Geometry check sheet. Reference: the model listing, model coordinates, mm. A direction names the side the tool comes from. Give positions to 0.01 mm unless a question says otherwise; leave off trailing zeros. Write each loop counter-clockwise with the first axis right and the second up, starting at its lowest first coordinate (ties: lowest second). Pieces come first, ordered by that corner, then holes.
(1) Cross-section at B-B (y = 0). Record the boundary of the cut face in (x, z), and give its area (3 significant figures).
(2) Cross-section at C-C (z = 4.5). Record the boundary of the cut face in (x, y).
(3) Tool access check on faces 1 (the flat face through (124.627, -15, 25)), 2 (the flat face through (-2, 83.745, 25)). Record the directions out of +Z, -Z, +X, -X, +Y, -Y that give a thin tool (end or side, any length) a straight path to the whole face; none if there is none.
(4) Mould release check, pull along X, two halves, no side actions. Record for faces 3 (the flat face through (121.627, -12, 25)), 4 (the flat face through (-125.373, -12, 25)), 5 (the flat face through (-2, -110.255, 25)), 6 (the flat face through (1, 86.745, 25)): +X half, -X half, draft (parallel to the pull), parting line (faces both ways), or undercut.
(5) Thickness scan on line 1 along X through (y, z) = (-99.5, 46); line 2 along Y through (x, z) = (18, 35). Record the ranges inside material, lowest first.
(6) Cross-section at A-A (x = -89). Record the boundary of the cut face in (y, z).
```python
from build123d import *

# Parameters (mm, degrees)
F0_W     = 3
F0_H     = 97
F0_H_2   = 3
F0_W_2   = 122
F0_W_3   = 115.3171807528
F0_W_4   = 6.6828192472
F0_W_5   = 244
F1_DEPTH = 50


with BuildPart() as f1:
    # F0 (on Top) → F1 (new body)
    with BuildSketch(Plane.XY):
        with Locations((-123.8728196025, 35.2448651371)):
            Rectangle(F0_W, F0_H)
        with Locations((-123.8728196025, 85.2448651371)):
            Rectangle(F0_W, F0_H_2)
        with Locations((-61.3728196025, 85.2448651371)):
            Rectangle(F0_W_2, F0_H_2)
        with Locations((57.2857707739, 85.2448651371)):
            Rectangle(F0_W_3, F0_H_2)
        with Locations((118.2857707739, 85.2448651371)):
            Rectangle(F0_W_4, F0_H_2)
        with Locations((123.1271803975, 85.2448651371)):
            Rectangle(F0_W, F0_H_2)
        Polygon((124.6271803975, 83.7448651371), (121.6271803975, 83.7448651371), (121.6271803975, -110.2551348629), (121.6271803975, -113.2551348629), (124.6271803975, -113.2551348629), align=None)
        with Locations((-0.3728196025, -111.7551348629)):
            Rectangle(F0_W_5, F0_H_2)
        with Locations((-123.8728196025, -61.7551348629)):
            Rectangle(F0_W, F0_H)
        with Locations((-123.8728196025, -111.7551348629)):
            Rectangle(F0_W, F0_H_2)
    extrude(amount=F1_DEPTH)


solid = f1.part
```
Reply:
1. outline: (-125.37, 0) - (-122.37, 0) - (-122.37, 50) - (-125.37, 50) - close; (121.63, 0) - (124.63, 0) - (124.63, 50) - (121.63, 50) - close
1. area: 300 mm2
2. outline: (-125.37, -113.26) - (124.63, -113.26) - (124.63, 86.74) - (-125.37, 86.74) - close; hole (-122.37, -110.26) - (121.63, -110.26) - (121.63, 83.74) - (-122.37, 83.74) - close
3. face 1: +Z, -Z, +X, +Y, -Y
3. face 2: +Z, -Z
4. face 3: undercut
4. face 4: -X half
4. face 5: undercut
4. face 6: draft
5. line 1: x = -125.37 to -122.37, 121.63 to 124.63
5. line 2: y = -113.26 to -110.26, 83.74 to 86.74
6. outline: (-113.26, 0) - (-110.26, 0) - (-110.26, 50) - (-113.26, 50) - close; (83.74, 0) - (86.74, 0) - (86.74, 50) - (83.74, 50) - close
